The model under review builds one solid part; all positions refer to its coordinate system, in mm. A direction names the side the tool comes from. Coordinates: 2 decimals unless noted, no trailing zeros. Order: outer loops, then holes, each group sorted by start corner. A loop starts at its lowest first (then second) coordinate and runs counter-clockwise, first axis right, second up.
```python
from build123d import *

# Parameters (mm, degrees)
ESBO_O1_W                = 30
ESBO_O1_H                = 10
RESSALTO_EXTRUS_O1_DEPTH = 20
ESBO_O2_R                = 5
CORTE_EXTRUS_O1_DEPTH    = 41


with BuildPart() as part:
    # Esboço1 → Ressalto-extrusão1 (new body)
    with BuildSketch(Plane.XY):
        Polygon((-40, 70), (-50, 70), (-50, 0), (0, 0), (0, 70), (-10, 70), (-10, 40), (-40, 40), align=None)
        with Locations((-25, 25)):
            Rectangle(ESBO_O1_W, ESBO_O1_H, mode=Mode.SUBTRACT)
    extrude(amount=RESSALTO_EXTRUS_O1_DEPTH)

    # Esboço2 → Corte-extrusão1 (cut, through all)
    with BuildSketch(Plane(origin=(0, 40, 0), x_dir=(1, 0, 0), z_dir=(0, 1, 0))):
        with Locations(Location((-25, -10, 0), (0, 0, 180))):  # turned: the seam where the file's is
            Circle(ESBO_O2_R)
    extrude(amount=-CORTE_EXTRUS_O1_DEPTH, mode=Mode.SUBTRACT)


solid = part.part
```
(1) We need section B-B, the plane y = 23. Write out the cut boundary in (x, z), and give its area (3 significant figures).
A:
outline: (-50, 0) - (-40, 0) - (-40, 20) - (-50, 20) - close; (-10, 0) - (0, 0) - (0, 20) - (-10, 20) - close
area: 400 mm2
(2) We need section C-C, the plane x = -25. Write out the cut boundary in (y, z).
A:
outline: (0, 0) - (20, 0) - (20, 5) - (0, 5) - close; (0, 15) - (20, 15) - (20, 20) - (0, 20) - close; (30, 0) - (40, 0) - (40, 5) - (30, 5) - close; (30, 15) - (40, 15) - (40, 20) - (30, 20) - close
(3) Draft analysis for pull direction X (two halves, no side actions). For faces 4 (the face through (-50, 35, 10)), 5 (the face through (-25, 35, 20)), 6 (the face through (-40, 25, 10)), state which applies: released by +X, released by -X, zero draft, split by the parting line, or undercut.
A:
face 4: released by -X
face 5: zero draft
face 6: undercut
(4) We need section D-D, the plane z = 2.25. Write out the cut boundary in (x, y), and give its area (3 significant figures).
A:
outline: (-50, 0) - (0, 0) - (0, 70) - (-10, 70) - (-10, 40) - (-40, 40) - (-40, 70) - (-50, 70) - close; hole (-40, 20) - (-10, 20) - (-10, 30) - (-40, 30) - close
area: 2,300 mm2
(5) Machinability: for faces 1 (the face through (-10, 25, 10)), 2 (the face through (-10, 55, 10)), 3 (the face through (-20, 10, 10)), which of the approach directions +Z, -Z, +X, -X, +Y, -Y give a long, thin tool a straight path to every point of the face, cutting with its end or side? Answer none if there is none.
A:
face 1: +Z, -Z
face 2: +Z, -Z, +Y
face 3: +Y, -Y
(6) We need section A-A, the plane z = 10. Write out the cut boundary in (x, y), and give its area (3 significant figures).
A:
outline: (-50, 0) - (-30, 0) - (-30, 20) - (-40, 20) - (-40, 30) - (-30, 30) - (-30, 40) - (-40, 40) - (-40, 70) - (-50, 70) - close; (-20, 0) - (0, 0) - (0, 70) - (-10, 70) - (-10, 40) - (-20, 40) - (-20, 30) - (-10, 30) - (-10, 20) - (-20, 20) - close
area: 2,000 mm2
(7) For pin 1 Ø6 at (y, z) = (19.5, 4) entering from +X; pin 2 Ø4 at (x, z) = (-33.5, 11.5) entering from +Y, all flat-tipped, find the tip position at first contact; note any pin that passes through.
A:
pin 1: stops at x = 0
pin 2: stops at y = 40
(8) Wall thickness on probe 1 along X at (y, z) = (60, 12); probe 2 along Z at (x, y) = (-25, 32.5); probe 3 along X at (y, z) = (13, 10.25): over which ranges is each line inside the solid? List them lowest first.
A:
probe 1: x = -50 to -40, -10 to 0
probe 2: z = 0 to 5, 15 to 20
probe 3: x = -50 to -29.99, -20.01 to 0
